from build123d import *

# Parameters (mm, degrees)
F0_W     = 5.5582858622
F0_H     = 21.6480456293
F0_W_2   = 7.0209950209
F0_H_2   = 43.2960875332
F0_H_3   = 18.7226310372
F1_DEPTH = 25.4
F3_W     = 95.0758680701
F3_H     = 67.8695440292
F3_W_2   = 21.9405852258
F3_H_2   = 22.2331248224
F4_DEPTH = 25.4


with BuildPart() as f1:
    # F0 (on Front) → F1 (new body)
    with BuildSketch(Plane.XZ):
        Polygon((-37.8840751946, 33.3496890962), (-75.9144276381, 33.3496890962), (-75.9144276381, -33.3496890962), (-5.5582858622, -33.3496890962), (-5.5582858622, -11.7016434669), (0, -11.7016434669), (0, -33.3496890962), (31.740706414, -33.3496890962), (31.740706414, 9.946398437), (38.7617014349, 9.946398437), (38.7617014349, -33.3496890962), (75.9144276381, -33.3496890962), (75.9144276381, 33.3496890962), (25.3048082814, 33.3496890962), (25.3048082814, -9.3613192439), (-37.8840751946, -9.3613192439), align=None)
        Polygon((-37.8840751946, 76.0606974363), (-37.8840751946, 33.3496890962), (-21.5017739683, 33.3496890962), (-21.5017739683, 56.1678977683), (8.9225070551, 56.1678977683), (8.9225070551, 33.3496890962), (25.3048082814, 33.3496890962), (25.3048082814, 76.0606974363), align=None)
        Polygon((-21.5017739683, 33.3496890962), (-37.8840751946, 33.3496890962), (-37.8840751946, -9.3613192439), (25.3048082814, -9.3613192439), (25.3048082814, 33.3496890962), (8.9225070551, 33.3496890962), (8.9225070551, 10.5314804241), (-21.5017739683, 10.5314804241), align=None)
        with Locations((-2.7791429311, -22.5256662816)):
            Rectangle(F0_W, F0_H)
        with Locations((-2.7791429311, -44.1737119108)):
            Rectangle(F0_W, F0_H)
        with Locations((35.2512039244, -11.7016453296)):
            Rectangle(F0_W_2, F0_H_2)
        with Locations((35.2512039244, -42.7110046148)):
            Rectangle(F0_W_2, F0_H_3)
    extrude(amount=F1_DEPTH)

    # F3 (on face) → F4 (join)
    with BuildSketch(Plane.XZ.offset(25.4)):
        Rectangle(F3_W, F3_H)
        with Locations((-10.9702926129, 11.1165624112)):
            Rectangle(F3_W_2, F3_H_2, mode=Mode.SUBTRACT)
    extrude(amount=F4_DEPTH)


solid = f1.part
The model under review builds one solid part; all positions refer to its coordinate system, in mm. A direction names the side the tool comes from. Coordinates: 2 decimals unless noted, no trailing zeros. Loops run counter-clockwise (first coordinate to the right, second up) from the corner with the lowest first, then second, coordinate; pieces in that order, holes last.
(1) Tool access review of faces 5 (the flat face through (-11, -25.4, 6)), 6 (the flat face through (-7, -13, 56.168)), 7 (the flat face through (-57, -13, 33.35)): name each direction out of +Z, -Z, +X, -X, +Y, -Y from which nothing blocks a thin tool from reaching the whole face with its end or side.
Determined:
face 5: -Y
face 6: +Y, -Y
face 7: +Z, -X, +Y
(2) Consider section A-A, the plane x = -19.5. Give the boundary of the cut face in (y, z).
Determined:
outline: (-50.8, -33.93) - (-25.4, -33.93) - (-25.4, -33.35) - (0, -33.35) - (0, 10.53) - (-25.4, 10.53) - (-25.4, 0) - (-50.8, 0) - close; (-50.8, 22.23) - (-25.4, 22.23) - (-25.4, 33.93) - (-50.8, 33.93) - close; (-25.4, 56.17) - (0, 56.17) - (0, 76.06) - (-25.4, 76.06) - close
(3) Consider section B-B, the plane y = -6.5. Give the boundary of the cut face in (x, z), plus the area to 3 significant figures.
Determined:
outline: (-75.91, -33.35) - (-5.56, -33.35) - (-5.56, -55) - (0, -55) - (0, -33.35) - (31.74, -33.35) - (31.74, -52.07) - (38.76, -52.07) - (38.76, -33.35) - (75.91, -33.35) - (75.91, 33.35) - (25.3, 33.35) - (25.3, 76.06) - (-37.88, 76.06) - (-37.88, 33.35) - (-75.91, 33.35) - close; hole (-21.5, 10.53) - (8.92, 10.53) - (8.92, 56.17) - (-21.5, 56.17) - close
area: 11,700 mm2
(4) Consider section C-C, the plane z = -8. Give the boundary of the cut face in (x, y).
Determined:
outline: (-75.91, -25.4) - (-47.54, -25.4) - (-47.54, -50.8) - (47.54, -50.8) - (47.54, -25.4) - (75.91, -25.4) - (75.91, 0) - (-75.91, 0) - close
(5) Consider section D-D, the plane z = 14.5. Give the boundary of the cut face in (x, y), plus the area to 3 significant figures.
Determined:
outline: (-75.91, -25.4) - (-47.54, -25.4) - (-47.54, -50.8) - (-21.94, -50.8) - (-21.94, -25.4) - (-21.5, -25.4) - (-21.5, 0) - (-75.91, 0) - close; (0, -50.8) - (47.54, -50.8) - (47.54, -25.4) - (75.91, -25.4) - (75.91, 0) - (8.92, 0) - (8.92, -25.4) - (0, -25.4) - close
area: 4,940 mm2
(6) Insertion check: P1, Ø10, axis at y = -45, z = -3.5, coming from the -X side; P2, Ø24, axis at x = -12, y = -36.5, coming from the -Z side; P3, Ø14, axis at x = -68.5, z = -7, coming from the -Y side; P4, Ø0.5, axis at x = -28.5, z = -33.5, coming from the +Y side. Each pin has a flat end and moves straight along its axis. Give the tip position at first contact, or say it passes through.
Determined:
P1: stops at x = -47.54
P2: stops at z = -33.93
P3: stops at y = -25.4
P4: stops at y = 0
(7) Draft analysis for pull direction Z (two halves, no side actions). For faces 1 (the flat face through (-62, -25.4, 0)), 2 (the flat face through (0, -38, 11)), 3 (the flat face through (-11, -38, 22.233)), 4 (the flat face through (16, -13, -33.35)), state which applies: +Z half, -Z half, draft (parallel to the pull), parting line (faces both ways), or undercut.
Determined:
face 1: draft
face 2: undercut
face 3: undercut
face 4: -Z half
(8) Wall thickness on L1, parallel to X at y = -25, z = 11.5; L2, parallel to X at y = -42, z = 16.5; L3, parallel to Y at x = 19.5, z = 66: over which ranges is each line inside the solid? List them lowest first.
Determined:
L1: x = -75.91 to -21.5, 8.92 to 75.91
L2: x = -47.54 to -21.94, 0 to 47.54
L3: y = -25.4 to 0
